from build123d import *

# Parameters (mm, degrees)
F0_R     = 9.5
F0_R_2   = 5
F1_DEPTH = 29
F2_R     = 0.25
F3_W     = 3
F3_H     = 1.5


with BuildPart() as f1:
    # F0 (on Top) → F1 (new body)
    with BuildSketch(Plane.XY):
        Circle(F0_R)
        Circle(F0_R_2, mode=Mode.SUBTRACT)
    extrude(amount=F1_DEPTH)

    # F2
    f2_edges = [f1.edges().sort_by_distance(p)[0] for p in [
        (-9.5, 0, 29),
        (-5, 0, 29),
        (-9.5, 0, 0),
        (-5, 0, 0),
    ]]
    fillet(f2_edges, radius=F2_R)

    # F3 (on Front) → F4 (revolve, cut)
    with BuildSketch(Plane.XZ):
        with Locations((10, 24.25)):
            Rectangle(F3_W, F3_H)
        with Locations((10, 4.75)):
            Rectangle(F3_W, F3_H)
    revolve(axis=Axis((0, 0, 23.490791), (0, 0, 1)), mode=Mode.SUBTRACT)


solid = f1.part
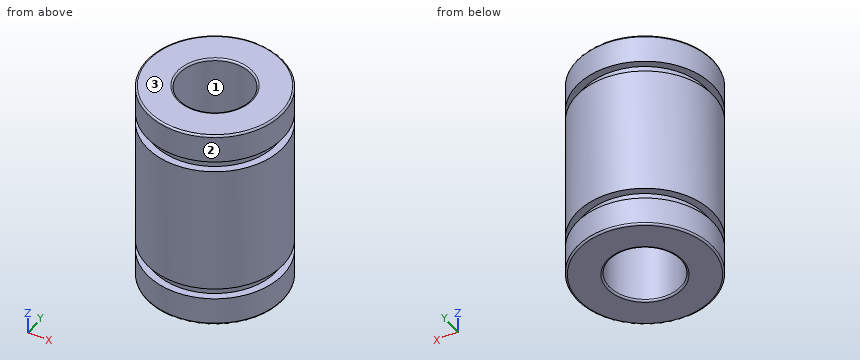
Here's how the part is built. I have some questions about the finished solid (model axes, mm). Face numbers are marked on the shaded views. Coordinates: 2 decimals unless noted, no trailing zeros. Order: outer loops, then holes, each group sorted by start corner. A loop starts at its lowest first (then second) coordinate and runs counter-clockwise, first axis right, second up. Notation, with made-up numbers: (-25, -22) -> (34, -22) arc R24 ccw to (34, 9) -> close; hole circle Ø2 at (16, 45.25). An arc over 180 degrees is marked (long way). Answer in a Markdown table with one row per item.
(1) Will these pins go through, and if not, where does the flat tip stop? pin 1 Ø2 at (x, z) = (4, 8.5) entering from +Y; pin 2 Ø10 at (x, z) = (-6.5, 18) entering from -Y; pin 3 Ø1.5 at (x, y) = (-3.5, -0.5) entering from -Z; pin 4 Ø5.5 at (x, y) = (-0.5, -4) entering from -Z.
Answer key:
| item | result |
|---|---|
| pin 1 | y = 9.01 |
| pin 2 | y = -9.38 |
| pin 3 | through |
| pin 4 | z = 0 |
(2) Thinking about a two-plate mould opening in X: for the marked faces 1, 2 and 3, which applies, +X half, -X half, draft (parallel to the pull), parting line (faces both ways), or undercut?
Answer key:
| item | result |
|---|---|
| face 1 | undercut |
| face 2 | parting line |
| face 3 | draft |
(3) I want a section at C-C on z = 13.5. List the corners of the cut face in (x, y) for me.
Answer key:
| item | result |
|---|---|
| outline | circle Ø19 at (0, 0); hole circle Ø10 at (0, 0) |
(4) Please list where these lines run through material, in increasing order: probe 1 along Z at (x, y) = (-7.25, -5.5); probe 2 along Y at (x, z) = (0, 6.5); probe 3 along X at (y, z) = (0.25, 24).
Answer key:
| item | result |
|---|---|
| probe 1 | 0 to 4, 5.5 to 23.5, 25 to 29 |
| probe 2 | -9.5 to -5, 5 to 9.5 |
| probe 3 | -8.5 to -4.99, 4.99 to 8.5 |
